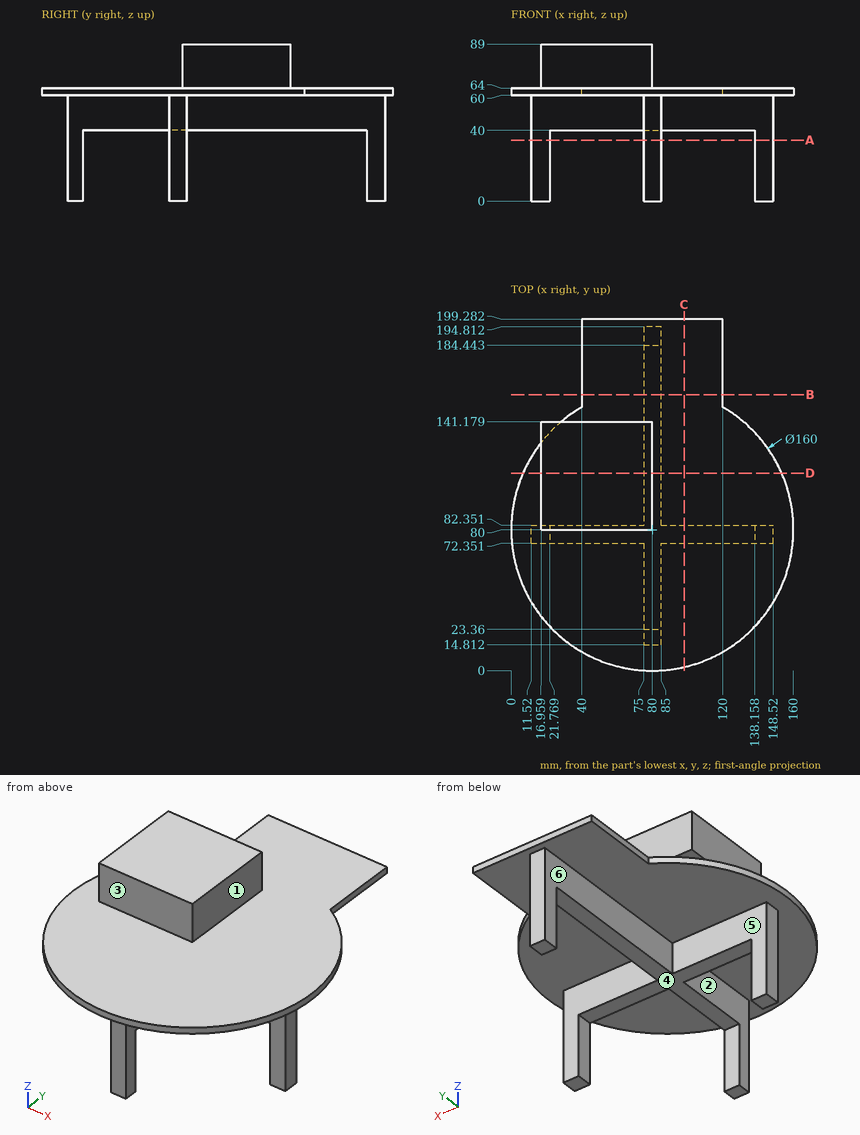
For this review, use the dimensioned drawing (mm, ordinates from the lowest corner) and the shaded views. A direction names the side the tool comes from. Give positions to 0.01 mm unless a question says otherwise; leave off trailing zeros. Order: outer loops, then holes, each group sorted by start corner. A loop starts at its lowest first (then second) coordinate and runs counter-clockwise, first axis right, second up. Notation, with made-up numbers: (21.25, 67.25) - (73.25, 67.25) arc R18 cw to (73.25, 84.25) - close; hole circle Ø4 at (51.5, 68). An arc over 180 degrees is marked (long way). Use CSV: the item, a comma, the result in double quotes. Start each with the question number.
Q1. Draft analysis for pull direction Y (two halves, no side actions). For the marked faces 4, 5 and 6, state which applies: pulls with the +Y half, pulls with the -Y half, needs draft (parallel to the pull), parting line crosses it, or undercut.
Q2. Take a section at B-B (y = 156.5). State the section outline as (x, z) points.
Q3. For P1, Ø20, axis at y = 98.5, z = 70.5, coming from the -X side; P2, Ø5, axis at y = 79, z = 18.5, coming from the +X side; P3, Ø10, axis at x = 67, z = 19.5, coming from the +Y side; P4, Ø9, axis at x = 25.5, y = 137, coming from the -Z side, all flat-tipped, find the tip position at first contact; note any pin that passes through.
Q4. Take a section at C-C (x = 98). State the section outline as (y, z) points.
Q5. Take a section at D-D (y = 112). State the section outline as (x, z) points.
Q6. Take a section at A-A (z = 34.5). State the section outline as (x, y) points, and give its area (3 significant figures).
Q7. For line 1 (X direction, y = 82, z = 18.5); line 2 (X direction, y = 148.5, z = 45); line 3 (Z direction, x = 68, y = 173), list the stretches that pass through material, from the lowest coordinate up.
Q8. Machinability: for the marked faces 1, 2 and 3, which of the approach directions +Z, -Z, +X, -X, +Y, -Y give a long, thin tool a straight path to every point of the face, cutting with its end or side? Answer none if there is none.
Calculated:
1,face 4,"undercut"
1,face 5,"pulls with the +Y half"
1,face 6,"needs draft"
2,outline,"(40, 60) - (75, 60) - (75, 40) - (85, 40) - (85, 60) - (120, 60) - (120, 64) - (40, 64) - close"
3,P1,"stops at x = 0.75"
3,P2,"stops at x = 148.52"
3,P3,"passes through"
3,P4,"stops at z = 60"
4,outline,"(2.05, 60) - (72.35, 60) - (72.35, 40) - (82.35, 40) - (82.35, 60) - (199.28, 60) - (199.28, 64) - (2.05, 64) - close"
5,outline,"(6.68, 60) - (75, 60) - (75, 40) - (85, 40) - (85, 60) - (153.32, 60) - (153.32, 64) - (80, 64) - (80, 89) - (16.96, 89) - (16.96, 64) - (6.68, 64) - close"
6,outline,"(11.52, 72.35) - (21.77, 72.35) - (21.77, 82.35) - (11.52, 82.35) - close; (75, 14.81) - (85, 14.81) - (85, 23.36) - (75, 23.36) - close; (75, 184.44) - (85, 184.44) - (85, 194.81) - (75, 194.81) - close; (138.16, 72.35) - (148.52, 72.35) - (148.52, 82.35) - (138.16, 82.35) - close"
6,area,"395 mm²"
7,line 1,"x = 11.52 to 21.77, 138.16 to 148.52"
7,line 2,"x = 75 to 85"
7,line 3,"z = 60 to 64"
8,face 1,"+Z, +X, +Y, -Y"
8,face 2,"-Z, -X, -Y"
8,face 3,"+Z, +X, -X, -Y"
